Read the model definition and answer for the solid it produces. Units are mm, in the model's axes. A direction names the side the tool comes from. Coordinates: 2 decimals unless noted, no trailing zeros. Loops run counter-clockwise (first coordinate to the right, second up) from the corner with the lowest first, then second, coordinate; pieces in that order, holes last. Notation, with made-up numbers: M 81.25,71.25 L 124.25,71.25 A32 ccw 124.25,107.25 Z; hole C 35.25,-17 d9. An arc over 180 degrees is marked long. Use one line per item in the form item = value. Start each with the question number.
1. The part is cut by section A-A (y = 2.05). Give the vertices of the cut face in (x, z), plus the area to 3 significant figures.
2. The part is cut by section B-B (x = 0). Give the number of separate pieces and of enclosed holes in the cut face, plus the area to 3 significant figures.
3. Flat-ended cylindrical pins translate along their axes: pin 1 (1 mm diameter, centred on x = 4.5, y = 0.5, fed in from +Z); pin 2 (4 mm diameter, centred on x = 1.5, z = 7, fed in from +Y); pin 3 (1.8 mm diameter, centred on x = 0, z = 0, fed in from +Y); pin 4 (1.5 mm diameter, centred on x = 2.5, y = 2, fed in from -Z). Find the tip coordinate at first contact, or state that the pin passes through.
4. For a pull along Z with two mould halves and no side action, classify faces 1 (the cylindrical face through (-6, 1, 0)), 2 (the cylindrical face through (-9.76, 1.23, -2.17)), 3 (the cylindrical face through (0.45, 1.18, 1.43)), 4 (the flat face through (-2, 0, 0)) as released by +Z, released by -Z, zero draft, split by the parting line, or undercut.
5. A tool of negligible diameter and unlimited length cuts with its end or side. For faces 5 (the flat face through (-3, 4.5, 2)), 6 (the cylindrical face through (0.9, 3.49, 2.86)), from which of +Z, -Z, +X, -X, +Y, -Y can it reach the whole face along a straight path? Write none if from no direction.
6. Find the intervals of material crossed by probe 1 along X at (y, z) = (1.15, 6.5); probe 2 along Y at (x, z) = (-5, -6.5); probe 3 along Z at (x, y) = (-6.25, 1.1), in increasing order. Write a range as [from, to].
from build123d import *

# Parameters (mm, degrees)
SKETCH_1_R      = 10
SKETCH_1_R_2    = 1.5
SKETCH_1_R_3    = 1
EXTRUDE_1_DEPTH = 2.5
SKETCH_2_R      = 4.5
SKETCH_2_R_2    = 3
EXTRUDE_2_DEPTH = 2
CHAMFER_1_SIZE  = 0.1
CHAMFER_2_SIZE  = 0.1


with BuildPart() as part:
    # 草图1 → 凸台-拉伸1 (new body)
    with BuildSketch(Plane(origin=(0, 0, 0), x_dir=(1, 0, 0), z_dir=(0, 1, 0))):
        with Locations(Location((0, 0, 0), (0, 0, 270))):
            Circle(SKETCH_1_R)
        with Locations(Location((0, 0, 0), (0, 0, 270))):
            Circle(SKETCH_1_R_2, mode=Mode.SUBTRACT)
        with Locations(Location((0, 7, 0), (0, 0, 270))):
            Circle(SKETCH_1_R_3, mode=Mode.SUBTRACT)
        with Locations(Location((7, 0, 0), (0, 0, 270))):
            Circle(SKETCH_1_R_3, mode=Mode.SUBTRACT)
        with Locations(Location((0, -7, 0), (0, 0, 270))):
            Circle(SKETCH_1_R_3, mode=Mode.SUBTRACT)
        with Locations(Location((-7, 0, 0), (0, 0, 270))):
            Circle(SKETCH_1_R_3, mode=Mode.SUBTRACT)
    extrude(amount=EXTRUDE_1_DEPTH)

    # 草图2 → 凸台-拉伸2 (add)
    with BuildSketch(Plane(origin=(0, 2.5, 0), x_dir=(1, 0, 0), z_dir=(0, 1, 0))):
        with Locations(Location((0, 0, 0), (0, 0, 270))):
            Circle(SKETCH_2_R)
        with Locations(Location((0, 0, 0), (0, 0, 270))):
            Circle(SKETCH_2_R_2, mode=Mode.SUBTRACT)
    extrude(amount=EXTRUDE_2_DEPTH)

    # 倒角1
    chamfer_1_edges = [part.edges().sort_by_distance(p)[0] for p in [
        (0, 4.5, -4.5),
    ]]
    chamfer(chamfer_1_edges, length=CHAMFER_1_SIZE)

    # 倒角2
    chamfer_2_edges = [part.edges().sort_by_distance(p)[0] for p in [
        (0, 0, -10),
        (0, 2.5, -4.5),
        (0, 2.5, -3),
        (0, 4.5, -3),
        (0, 2.5, -10),
        (0, 2.5, -1.5),
    ]]
    chamfer(chamfer_2_edges, length=CHAMFER_2_SIZE)


solid = part.part
Computed values:
q1.outline = C 0,0 d20; hole C -7,0 d2; hole C 0,0 d3; hole C 0,-7 d2; hole C 0,7 d2; hole C 7,0 d2
q1.area = 295 mm²
q2.separate_pieces = 4
q2.enclosed_holes = 0
q2.area = 38.5 mm²
q3.pin_1 = 9.17
q3.pin_2 = 2.5
q3.pin_3 = through
q3.pin_4 = -9.85
q4.face_1 = undercut
q4.face_2 = split by the parting line
q4.face_3 = undercut
q4.face_4 = zero draft
q5.face_5 = +Z, -Z, +X, -X, +Y
q5.face_6 = +Y
q6.probe_1 = [-7.6, -0.87], [0.87, 7.6]
q6.probe_2 = [0, 2.5]
q6.probe_3 = [-7.81, -0.66], [0.66, 7.81]
